from build123d import *

# Parameters (mm, degrees)
SALIENTE_EXTRUIR1_DEPTH    = 15
CORTAR_EXTRUIR1_DEPTH      = 10
CORTAR_EXTRUIR1_DEPTH_BACK = 39
VACIADO1_T                 = -2
SALIENTE_EXTRUIR2_DEPTH    = 10
CORTAR_EXTRUIR2_DEPTH      = 39
CROQUIS9_R                 = 1.45
CORTAR_EXTRUIR3_DEPTH      = 33
CORTAR_EXTRUIR4_DEPTH      = 12
CROQUIS11_W                = 2
CROQUIS11_H                = 8
CORTAR_EXTRUIR5_DEPTH      = 2
CROQUIS14_R                = 3
SALIENTE_EXTRUIR3_DEPTH    = 8
CROQUIS15_R                = 1.45
CORTAR_EXTRUIR6_DEPTH      = 8


with BuildPart() as part:
    # Croquis1 → Saliente-Extruir1 (new body)
    with BuildSketch(Plane.XY):
        Polygon((0, 0), (0, 33), (63, 33), (63, 0), (63, -6), (0, -6), align=None)
    extrude(amount=SALIENTE_EXTRUIR1_DEPTH)

    # Croquis2 → Cortar-Extruir1 (cut, two sides: drawn at the far end of the back side and taken through both)
    with BuildSketch(Plane.XZ.offset(6).offset(-CORTAR_EXTRUIR1_DEPTH_BACK)):
        Polygon((0, 15), (0, 6), (18, 15), align=None)
        Polygon((63, 15), (63, 6), (45, 15), align=None)
    extrude(amount=CORTAR_EXTRUIR1_DEPTH + CORTAR_EXTRUIR1_DEPTH_BACK, mode=Mode.SUBTRACT)

    # Vaciado1
    vaciado1_openings = [part.faces().sort_by_distance(p)[0] for p in [
        (31.5, 13.5, 0),
    ]]
    offset(amount=VACIADO1_T, openings=vaciado1_openings, kind=Kind.INTERSECTION)

    # Croquis3 → Saliente-Extruir2 (add)
    with BuildSketch(Plane(origin=(0, 0, 0), x_dir=(-1, 0, 0), z_dir=(0, 0, -1))):
        with BuildLine():
            Line((-63, 30), (-63, 27.354248689))
            ThreePointArc((-63, 27.354248689), (-58.125593258, 26.466361738), (-56.127016654, 31))
            Line((-56.127016654, 31), (-57.171572875, 31))
            ThreePointArc((-57.171572875, 31), (-60.507305936, 32.956795679), (-63, 30))
        make_face()
        with BuildLine():
            Line((-6.872983346, 31), (-5.828427125, 31))
            ThreePointArc((-5.828427125, 31), (-0.878679656, 32.121320344), (-2, 27.171572875))
            Line((-2, 27.171572875), (-2, 26.127016654))
            ThreePointArc((-2, 26.127016654), (-5.828427125, 27.171572875), (-6.872983346, 31))
        make_face()
    extrude(amount=-SALIENTE_EXTRUIR2_DEPTH)

    # Croquis8 → Cortar-Extruir2 (cut)
    with BuildSketch(Plane.XZ.offset(6)):
        Polygon((0, 6), (0, 18.606217888), (63, 18.606217888), (63, 6), (45, 15), (18, 15), align=None)
    extrude(amount=-CORTAR_EXTRUIR2_DEPTH, mode=Mode.SUBTRACT)

    # Croquis9 → Cortar-Extruir3 (cut)
    with BuildSketch(Plane(origin=(0, 0, 0), x_dir=(-1, 0, 0), z_dir=(0, 0, -1))):
        with Locations((-60, 30)):
            Circle(CROQUIS9_R)
        with Locations((-3, 30)):
            Circle(CROQUIS9_R)
    extrude(amount=-CORTAR_EXTRUIR3_DEPTH, mode=Mode.SUBTRACT)

    # Croquis10 → Cortar-Extruir4 (cut)
    with BuildSketch(Plane.XY.offset(15)):
        with BuildLine():
            Line((6, 30), (6, 33))
            Line((6, 33), (0, 33))
            Line((0, 33), (0, 27))
            Line((0, 27), (3, 27))
            ThreePointArc((3, 27), (5.121320344, 27.878679656), (6, 30))
        make_face()
        with BuildLine():
            Line((60, 27), (63, 27))
            Line((63, 27), (63, 33))
            Line((63, 33), (57, 33))
            Line((57, 33), (57, 30))
            ThreePointArc((57, 30), (57.878679656, 27.878679656), (60, 27))
        make_face()
    extrude(amount=-CORTAR_EXTRUIR4_DEPTH, mode=Mode.SUBTRACT)

    # Croquis11 → Cortar-Extruir5 (cut)
    with BuildSketch(Plane(origin=(0, 0, 0), x_dir=(-1, 0, 0), z_dir=(0, 0, -1))):
        with Locations((-62, 3)):
            Rectangle(CROQUIS11_W, CROQUIS11_H)
    extrude(amount=-CORTAR_EXTRUIR5_DEPTH, mode=Mode.SUBTRACT)

    # Croquis14 → Saliente-Extruir3 (add)
    with BuildSketch(Plane.XZ.offset(6)):
        with Locations((31.5, 12)):
            Circle(CROQUIS14_R)
    extrude(amount=-SALIENTE_EXTRUIR3_DEPTH)

    # Croquis15 → Cortar-Extruir6 (cut)
    with BuildSketch(Plane(origin=(0, 2, 0), x_dir=(1, 0, 0), z_dir=(0, 1, 0))):
        with Locations(Location((31.5, -12, 0), (0, 0, 270))):
            Circle(CROQUIS15_R)
    extrude(amount=-CORTAR_EXTRUIR6_DEPTH, mode=Mode.SUBTRACT)


solid = part.part
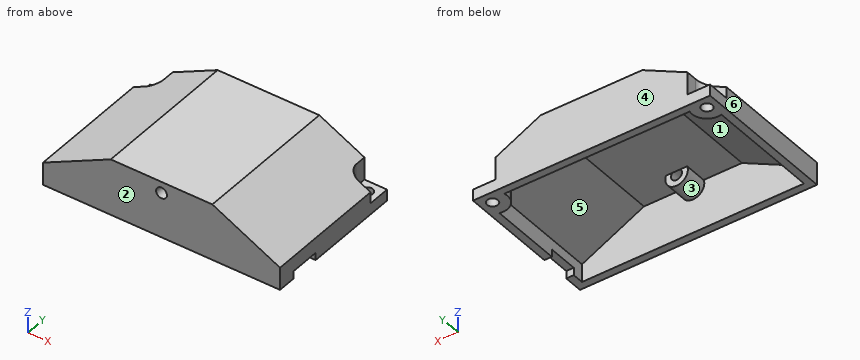
Geometry check sheet. Reference: the model listing, model coordinates, mm. Face numbers are marked on the shaded views. A direction names the side the tool comes from. Coordinates: 2 decimals unless noted, no trailing zeros. Order: outer loops, then holes, each group sorted by start corner. A loop starts at its lowest first (then second) coordinate and runs counter-clockwise, first axis right, second up. Notation, with made-up numbers: M 28,52 L 71,52 A25 ccw 71,75 Z; hole C 23,-34 d9. An arc over 180 degrees is marked long. Use CSV: the item, a comma, the result in double quotes.
Item 1: Tool access check on the marked faces 5 and 6. Record the directions out of +Z, -Z, +X, -X, +Y, -Y that give a thin tool (end or side, any length) a straight path to the whole face; none if there is none.
Returned:
face 5,"-Z"
face 6,"+Z, -Z, -X, +Y, -Y"
Item 2: Cross-section at A-A on x = 31.5. Record the cut outline in (y, z).
Returned:
outline,"M -6,0 L -4,0 L -4,9 L 2,9 L 2,10.55 L -6,10.55 Z; M -6,13.45 L 2,13.45 L 2,13 L 31,13 L 31,0 L 33,0 L 33,15 L -6,15 Z"
Item 3: Thickness scan on line 1 along Y through (x, z) = (60, 1.4); line 2 along Y through (x, z) = (25, 3.25); line 3 along X through (y, z) = (16, 1.75). Record the ranges inside material, lowest first.
Returned:
line 1,"y = -6 to -4, 26 to 28.55, 31.45 to 33"
line 2,"y = -6 to -4, 31 to 33"
line 3,"x = 0 to 2, 61 to 63"
Item 4: Cross-section at C-C on y = 0. Record the cut outline in (x, z).
Returned:
outline,"M 0,0 L 2,0 L 2,4.76 L 18.47,13 L 28.67,13 A3 ccw long 34.33,13 L 44.53,13 L 61,4.76 L 61,2 L 63,2 L 63,6 L 45,15 L 18,15 L 0,6 Z; hole C 31.5,12 d2.9"
Item 5: Mould release check, pull along Y, two halves, no side actions. Record for the marked faces 1, 2, 3 and 4: pulls with the +Y half, pulls with the -Y half, needs draft (parallel to the pull), parting line crosses it, or undercut.
Returned:
face 1,"undercut"
face 2,"pulls with the -Y half"
face 3,"undercut"
face 4,"pulls with the +Y half"
Item 6: Cross-section at B-B on y = 5.5. Record the cut outline in (x, z).
Returned:
outline,"M 0,0 L 2,0 L 2,4.76 L 18.47,13 L 44.53,13 L 61,4.76 L 61,2 L 63,2 L 63,6 L 45,15 L 18,15 L 0,6 Z"
Item 7: Cross-section at D-D on y = 14.5. Record the cut outline in (x, z), then the cut area to 3 significant figures.
Returned:
outline,"M 0,0 L 2,0 L 2,4.76 L 18.47,13 L 44.53,13 L 61,4.76 L 61,0 L 63,0 L 63,6 L 45,15 L 18,15 L 0,6 Z"
area,"152 mm2"
Item 8: Gauge pin test, flat ends, axial feed: pin 1 Ø3 at (x, y) = (29.5, 2) entering from -Z; pin 2 Ø3.5 at (y, z) = (32, 4.5) entering from -X; pin 3 Ø5 at (x, y) = (13, 27.5) entering from +Z; pin 4 Ø1.7 at (x, y) = (60, 30) entering from -Z. Record the tip position at first contact, or that the pin passes through.
Returned:
pin 1,"stops at z = 9.04"
pin 2,"stops at x = 0"
pin 3,"stops at z = 13.75"
pin 4,"passes through"
